CAD build for the part. Positions are in the model's coordinates, mm. Give positions to 0.01 mm unless a question says otherwise; leave off trailing zeros. Order: outer loops, then holes, each group sorted by start corner. A loop starts at its lowest first (then second) coordinate and runs counter-clockwise, first axis right, second up. Notation, with made-up numbers: (-30, -12.75) -> (-5, -12.75) arc R34 ccw to (-5, 18.25) -> close; hole circle Ø4 at (31, 4). An arc over 180 degrees is marked (long way). Use one line per item in the form item = value. Start each with the question number.
1) Probe line 1 (X direction, y = 8.25, z = 237.5); line 2 (X direction, y = 6.25, z = 437.5); line 3 (Y direction, x = 7.5, z = 268). List the from-to ranges inside material, lowest first.
2) Cut at A-A, the plane z = 300. Give the cut face in (x, y), and give its area (3 significant figures).
3) Drop flat-ended pins along their axis: P1, Ø3, axis at x = 12, z = 37, coming from the +Y side; P2, Ø2, axis at x = 11.12, z = 12.5, coming from the +Y side; P3, Ø1, axis at y = 10.5, z = 130, coming from the +X side. Give the stop position or say it passes through.
from build123d import *

# Parameters (mm, degrees)
EXTRUDE_1_DEPTH           = 450
HOLE_WIZARD_5_D           = 3.5
HOLE_WIZARD_5_CBORE_D     = 5.8
HOLE_WIZARD_5_CBORE_DEPTH = 4.5
HOLE_WIZARD_4_D           = 3.5
HOLE_WIZARD_4_CBORE_D     = 5.8
HOLE_WIZARD_4_CBORE_DEPTH = 4.5
HOLE_WIZARD_3_D           = 3.5
HOLE_WIZARD_3_DEPTH       = 7.916912277
HOLE_WIZARD_3_CBORE_D     = 5.8
HOLE_WIZARD_3_CBORE_DEPTH = 4.5


with BuildPart() as part:
    # 草图1 → 凸台-拉伸1 (new body)
    with BuildSketch(Plane.XY):
        Polygon((5.617628384, 4.221881307), (16.617628384, 4.221881307), (17.117628384, 4.721881307), (17.117628384, 8.221881307), (14.117628384, 9.445409037), (14.117628384, 9.987809251), (17.117628384, 11.343384147), (17.117628384, 11.721881307), (16.617628384, 12.221881307), (5.617628384, 12.221881307), (5.117628384, 11.721881307), (5.117628384, 11.211336981), (8.117628384, 9.987809251), (8.117628384, 9.445409037), (5.117628384, 8.221881307), (5.117628384, 4.721881307), align=None)
    extrude(amount=EXTRUDE_1_DEPTH)

    # 孔5 (through all)
    with Locations(Plane(origin=(11.117628384, 12.221881307, 12.5), x_dir=(0, 0, 1), z_dir=(0, 1, 0))):
        with Locations((0, 0), (25, 0), (50.00439355, 0), (75, 0), (100, 0), (125, 0), (150, 0), (175, 0), (200, 0), (225, 0), (250, 0), (275, 0), (300, 0), (325, 0), (350, 0), (375, 0), (400, 0), (425, 0)):
            CounterBoreHole(HOLE_WIZARD_5_D / 2, HOLE_WIZARD_5_CBORE_D / 2, HOLE_WIZARD_5_CBORE_DEPTH)

    # 孔4 (through all)
    with Locations(Plane(origin=(11.117628384, 12.221881307, 412.5), x_dir=(0, 0, 1), z_dir=(0, 1, 0))):
        with Locations((0, 0), (-25, 0), (-74.975489716, 0), (-75, 0), (-100, 0), (-150.000497417, 0), (-150, 0), (-175, 0), (-200, 0), (-225, 0), (-250, 0), (-275, 0), (-300, 0), (-325, 0), (-350, 0), (-375, 0)):
            CounterBoreHole(HOLE_WIZARD_4_D / 2, HOLE_WIZARD_4_CBORE_D / 2, HOLE_WIZARD_4_CBORE_DEPTH)

    # 孔3
    with Locations(Plane(origin=(11.117628384, 12.221881307, 387.223861755), x_dir=(0, 0, 1), z_dir=(0, 1, 0))):
        with Locations((0, 0)):
            CounterBoreHole(HOLE_WIZARD_3_D / 2, HOLE_WIZARD_3_CBORE_D / 2, HOLE_WIZARD_3_CBORE_DEPTH, depth=HOLE_WIZARD_3_DEPTH)


solid = part.part
Result:
q1.line_1 = 5.19 to 8.22, 14.02 to 17.05
q1.line_2 = 5.12 to 9.37, 12.87 to 17.12
q1.line_3 = 4.22 to 9.19, 10.24 to 12.22
q2.outline = (5.12, 4.72) -> (5.62, 4.22) -> (16.62, 4.22) -> (17.12, 4.72) -> (17.12, 8.22) -> (14.12, 9.45) -> (14.12, 9.99) -> (17.12, 11.34) -> (17.12, 11.72) -> (16.62, 12.22) -> (5.62, 12.22) -> (5.12, 11.72) -> (5.12, 11.21) -> (8.12, 9.99) -> (8.12, 9.45) -> (5.12, 8.22) -> close
q2.area = 84.7 mm²
q3.P1 = 7.72
q3.P2 = through
q3.P3 = 16.36
